Could you check a few things on this model? Use its own coordinates, in mm. Face numbers are marked on the shaded views. A direction names the side the tool comes from. Round coordinates to 2 decimals unless told otherwise and drop trailing zeros. Write each loop counter-clockwise with the first axis right and the second up, starting at its lowest first coordinate (ties: lowest second). Pieces come first, ordered by that corner, then holes. Notation, with made-up numbers: (79, -35.5) -> (104, -35.5) arc R14 ccw to (104, -20.5) -> close; hole circle Ø6 at (53.5, 61.5). An arc over 180 degrees is marked (long way). One line per question, with ' | ' between items. Start each with the question number.
1. Imagine slicing it at C-C, the plane x = 120.5. List the corners of the cut face in (y, z) for me.
2. Imagine slicing it at D-D, the plane y = 36. List the corners of the cut face in (x, z) for me, and give its area (3 significant figures).
3. Imagine slicing it at A-A, the plane y = 74. List the corners of the cut face in (x, z) for me, and give its area (3 significant figures).
4. For pin 1 Ø1.5 at (y, z) = (89, 10.5) entering from +X; pin 2 Ø8 at (x, z) = (57.5, 35.5) entering from +Y; pin 3 Ø13.5 at (x, y) = (76.5, 31.5) entering from +Z, each with a flat end and sliding along its axis, tell me the tip position at first contact or that it passes through.
5. Thinking about a two-plate mould opening in Y: for the marked faces 1, 2, 3 and 4, which applies, released by +Y, released by -Y, zero draft, split by the parting line, or undercut?
6. For the marked faces 5, 6, 7 and 8, which set-ups out of +Z, -Z, +X, -X, +Y, -Y let a thin tool reach every point of the face, with its end or its side?
7. If I drill on line 1 along X through (y, z) = (62, 38.5); line 2 along Z through (x, y) = (85, 25.5); line 3 along Y through (x, z) = (110, 9.5), over which ranges is the centre line in solid material (lowest first)? Write a range as [from, to].
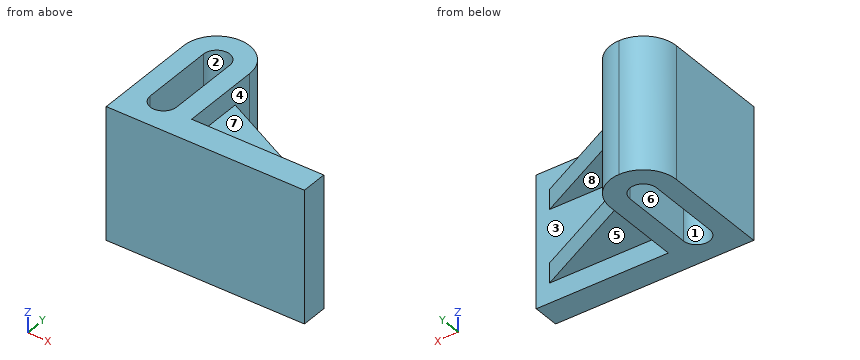
from build123d import *

# Parameters (mm, degrees)
BOSS_EXTRUDE1_DEPTH      = 50
BOSS_EXTRUDE1_DEPTH_BACK = 50
FILLET5_R                = 25
FILLET4_R                = 25
CUT_EXTRUDE1_DEPTH       = 209.62646045
BOSS_EXTRUDE2_START      = 20
BOSS_EXTRUDE2_DEPTH      = 15
BOSS_EXTRUDE3_START      = 40
BOSS_EXTRUDE3_DEPTH      = 15


with BuildPart() as part:
    # Sketch1 → Boss-Extrude1 (new, two sides: drawn at the far end of the back side and taken through both)
    with BuildSketch(Plane.XY.offset(-BOSS_EXTRUDE1_DEPTH_BACK)):
        Polygon((0, 0), (0, 105), (50, 105), (50, 20), (150, 20), (150, 0), align=None)
    extrude(amount=BOSS_EXTRUDE1_DEPTH + BOSS_EXTRUDE1_DEPTH_BACK)

    # Fillet5
    fillet5_edges = [part.edges().sort_by_distance(p)[0] for p in [
        (0, 105, 0),
    ]]
    fillet(fillet5_edges, radius=FILLET5_R)

    # Fillet4
    fillet4_edges = [part.edges().sort_by_distance(p)[0] for p in [
        (50, 105, 0),
    ]]
    fillet(fillet4_edges, radius=FILLET4_R - 0.0001)  # a hair under: the kernel refuses the full size

    # Sketch3 → Cut-Extrude1 (cut, through all)
    with BuildSketch(Plane.XY.offset(50)):
        with BuildLine():
            Line((35, 80), (35, 25))
            ThreePointArc((35, 25), (25, 15), (15, 25))
            Line((15, 25), (15, 80))
            ThreePointArc((15, 80), (25, 90), (35, 80))
        make_face()
    extrude(amount=-CUT_EXTRUDE1_DEPTH, mode=Mode.SUBTRACT)

    # Sketch5 → Boss-Extrude2 (add)
    with BuildSketch(Plane.XY.offset(BOSS_EXTRUDE2_START)):
        Polygon((50, 65), (140, 20), (50, 20), align=None)
    extrude(amount=BOSS_EXTRUDE2_DEPTH)

    # Sketch9 → Boss-Extrude3 (add)
    with BuildSketch(Plane(origin=(0, 0, 20), x_dir=(-1, 0, 0), z_dir=(0, 0, -1)).offset(BOSS_EXTRUDE3_START)):
        Polygon((-50, 20), (-50, 65), (-140, 20), align=None)
    extrude(amount=BOSS_EXTRUDE3_DEPTH)


solid = part.part
Geometry results:
1) outline: (0, -50) -> (20, -50) -> (20, -35) -> (29.75, -35) -> (29.75, -20) -> (20, -20) -> (20, 20) -> (29.75, 20) -> (29.75, 35) -> (20, 35) -> (20, 50) -> (0, 50) -> close
2) outline: (0, -50) -> (15, -50) -> (15, 50) -> (0, 50) -> close; (35, -50) -> (50, -50) -> (50, -35) -> (108, -35) -> (108, -20) -> (50, -20) -> (50, 20) -> (108, 20) -> (108, 35) -> (50, 35) -> (50, 50) -> (35, 50) -> close | area: 4,740 mm2
3) outline: (0, -50) -> (15, -50) -> (15, 50) -> (0, 50) -> close; (35, -50) -> (50, -50) -> (50, 50) -> (35, 50) -> close | area: 3,000 mm2
4) pin 1: stops at x = 48.6 | pin 2: stops at y = 63.23 | pin 3: stops at z = 35
5) face 1: undercut | face 2: undercut | face 3: released by +Y | face 4: zero draft
6) face 5: -Z, +X, +Y | face 6: +Z, -Z | face 7: +Z, +X, +Y | face 8: +X, +Y
7) line 1: x = [0, 15], [35, 50] | line 2: z = [-35, -20], [20, 35] | line 3: y = [0, 20]
